Drawing for the job (mm, zero at the part's lowest x, y, z). A direction names the side the tool comes from. Round coordinates to 2 decimals unless told otherwise and drop trailing zeros. Order: outer loops, then holes, each group sorted by start corner. A loop starts at its lowest first (then second) coordinate and runs counter-clockwise, first axis right, second up. Notation, with made-up numbers: (17.25, -19.75) - (31.25, -19.75) arc R18 cw to (31.25, 14.25) - close; hole circle Ø9 at (-28, 59.25). An arc over 180 degrees is marked (long way). Answer as a JSON object with one key per item and string values.
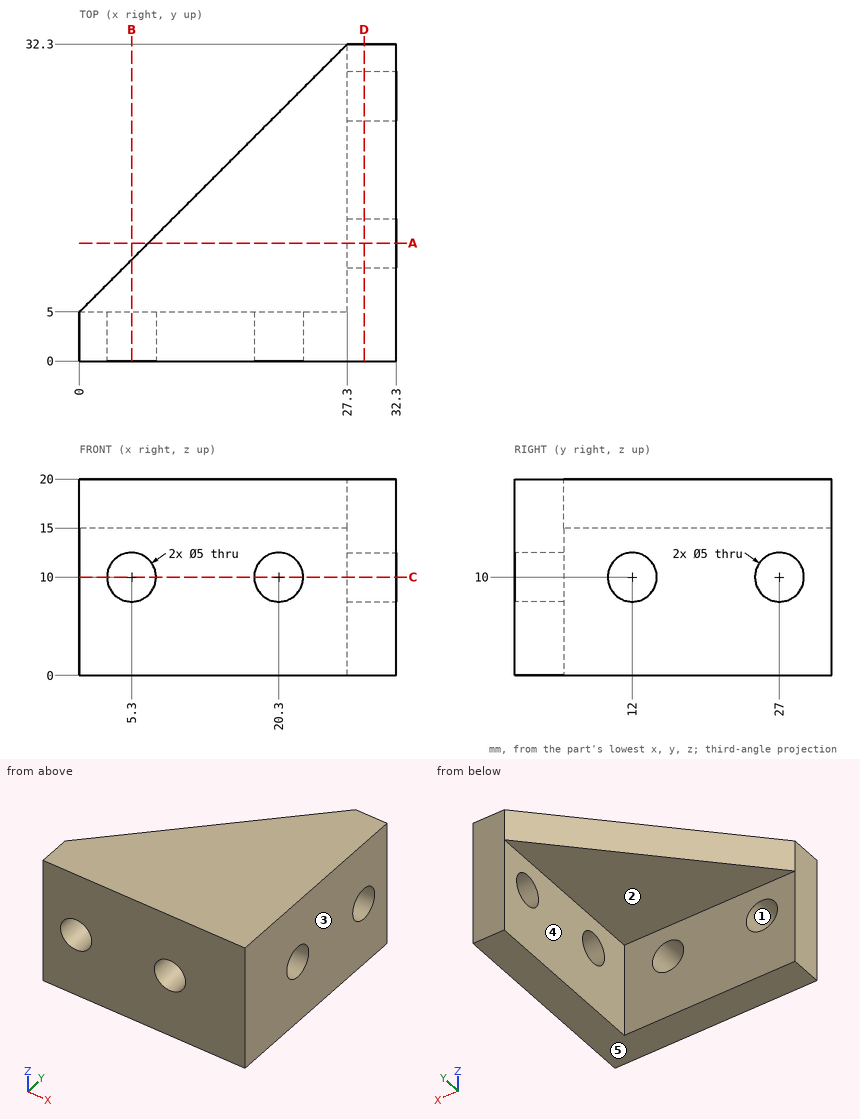
Item 1: Cut at D-D (x = 29). Write the cut outline in (y, z).
Taken from the geometry:
{"outline": "(0, 0) - (32.3, 0) - (32.3, 20) - (0, 20) - close; hole circle Ø5 at (12, 10); hole circle Ø5 at (27, 10)"}
Item 2: Tool access for the marked faces 4 and 5: list every direction of +Z, -Z, +X, -X, +Y, -Y with a clear straight run to the whole face (end or side of a thin tool).
Taken from the geometry:
{"face 4": "-Z, -X, +Y", "face 5": "-Z, +X, -X, +Y, -Y"}
Item 3: Cut at C-C (z = 10). Write the cut outline in (x, y), plus the area to 3 significant figures.
Taken from the geometry:
{"outline": "(0, 0) - (2.8, 0) - (2.8, 5) - (0, 5) - close; (7.8, 0) - (17.8, 0) - (17.8, 5) - (7.8, 5) - close; (22.8, 0) - (32.3, 0) - (32.3, 9.5) - (27.3, 9.5) - (27.3, 5) - (22.8, 5) - close; (27.3, 14.5) - (32.3, 14.5) - (32.3, 24.5) - (27.3, 24.5) - close; (27.3, 29.5) - (32.3, 29.5) - (32.3, 32.3) - (27.3, 32.3) - close", "area": "198 mm2"}
Item 4: Probe L1, parallel to X at y = 4, z = 10; L2, parallel to Y at x = 28.8, z = 10; L3, parallel to Z at x = 29.4, y = 27. List the from-to ranges inside material, lowest first. Write a range as from..to.
Taken from the geometry:
{"L1": "0..2.8, 7.8..17.8, 22.8..32.3", "L2": "0..9.5, 14.5..24.5, 29.5..32.3", "L3": "0..7.5, 12.5..20"}
Item 5: Cut at A-A (y = 12). Write the cut outline in (x, z).
Taken from the geometry:
{"outline": "(7, 15) - (27.3, 15) - (27.3, 12.5) - (32.3, 12.5) - (32.3, 20) - (7, 20) - close; (27.3, 0) - (32.3, 0) - (32.3, 7.5) - (27.3, 7.5) - close"}
Item 6: Cut at B-B (x = 5.3). Write the cut outline in (y, z), plus the area to 4 significant figures.
Taken from the geometry:
{"outline": "(0, 0) - (5, 0) - (5, 7.5) - (0, 7.5) - close; (0, 12.5) - (5, 12.5) - (5, 15) - (10.3, 15) - (10.3, 20) - (0, 20) - close", "area": "101.5 mm2"}
Item 7: Drop flat-ended pins along their axis: P1, Ø2, axis at x = 9, y = 11, coming from the -Z side; P2, Ø6, axis at x = 20.3, z = 10, coming from the +Y side; P3, Ø3, axis at y = 27, z = 10, coming from the +X side. Give the stop position or say it passes through.
Taken from the geometry:
{"P1": "z = 15", "P2": "y = 5", "P3": "through"}
Item 8: Two-plate mould, pull along X, no slides. Class the marked faces 1, 2 and 3: pulls with the +X half, pulls with the -X half, needs draft (parallel to the pull), parting line crosses it, or undercut.
Taken from the geometry:
{"face 1": "undercut", "face 2": "needs draft", "face 3": "pulls with the +X half"}
